Build history of the part. All positions in model axes, mm. A direction names the side the tool comes from. Coordinates: 2 decimals unless noted, no trailing zeros. Write each loop counter-clockwise with the first axis right and the second up, starting at its lowest first coordinate (ties: lowest second). Pieces come first, ordered by that corner, then holes.
```python
from build123d import *

# Parameters (mm, degrees)
F1_DEPTH = 5
F2_R     = 2.4
F2_R_2   = 0.75
F3_DEPTH = 2
F4_W     = 7
F4_H     = 3
F5_DEPTH = 3


with BuildPart() as f1:
    # F0 (on Right) → F1 (new body)
    with BuildSketch(Plane.YZ):
        with BuildLine():
            ThreePointArc((10, 30), (0, 40), (-10, 30))
            Line((-10, 30), (-10, 0))
            Line((-10, 0), (10, 0))
            Line((10, 0), (10, 30))
        make_face()
    extrude(amount=F1_DEPTH)

    # F2 (on face) → F3 (cut)
    with BuildSketch(Plane.YZ.offset(5)):
        with Locations((0, 30)):
            Circle(F2_R)
        with Locations((0, 30)):
            Circle(F2_R_2, mode=Mode.SUBTRACT)
    extrude(amount=-F3_DEPTH, mode=Mode.SUBTRACT)

    # F4 (on face) → F5 (join)
    with BuildSketch(Plane.YZ.offset(5)):
        with Locations((-6.5, -1.5)):
            Rectangle(F4_W, F4_H)
        with Locations((6.5, -1.5)):
            Rectangle(F4_W, F4_H)
    extrude(amount=-F5_DEPTH)


solid = f1.part
```
1. 3-axis set-ups, long thin cutter, end or side, ignore diameter. For faces 1 (the face through (4, -3, -2)), 2 (the face through (4.014, -0.098, 30.744)), 3 (the face through (5, 0, 19)), 4 (the face through (2, 6, -1)): which of +Z, -Z, +X, -X, +Y, -Y reach the whole face in a straight line?
Computed values:
face 1: -Z, +X, -X
face 2: +X
face 3: +Z, -Z, +X, +Y, -Y
face 4: -Z, -X, +Y, -Y
2. Saw through at B-B on y = 0. List the corners of the cut face in (x, z).
Computed values:
outline: (0, 0) - (5, 0) - (5, 27.6) - (3, 27.6) - (3, 29.25) - (5, 29.25) - (5, 30.75) - (3, 30.75) - (3, 32.4) - (5, 32.4) - (5, 40) - (0, 40) - close
3. Probe line 1 along Z through (x, y) = (3.2, 1.5); line 2 along Z through (x, y) = (4.1, 6.5); line 3 along Z through (x, y) = (1.25, 9). List the from-to ranges inside material, lowest first.
Computed values:
line 1: z = 0 to 28.13, 31.87 to 39.89
line 2: z = -3 to 37.6
line 3: z = 0 to 34.36
4. Saw through at D-D on z = 37.5. List the corners of the cut face in (x, y), plus the area to 3 significant figures.
Computed values:
outline: (0, -6.61) - (5, -6.61) - (5, 6.61) - (0, 6.61) - close
area: 66.1 mm2
5. Saw through at C-C on x = 0.5. List the corners of the cut face in (y, z), plus the area to 3 significant figures.
Computed values:
outline: (-10, 0) - (10, 0) - (10, 30) arc R10 ccw to (-10, 30) - close
area: 757 mm2
6. Saw through at A-A on x = 3.7. List the corners of the cut face in (y, z).
Computed values:
outline: (-10, -3) - (-3, -3) - (-3, 0) - (3, 0) - (3, -3) - (10, -3) - (10, 30) arc R10 ccw to (-10, 30) - close; circle Ø1.5 at (0, 30); hole circle Ø4.8 at (0, 30)
7. Flat gauge pins, fed straight in: pin 1 (6 mm diameter, centred on y = -1.5, z = 21.5, fed in from -X); pin 2 (0.9 mm diameter, centred on y = -7, z = -1.5, fed in from -X); pin 3 (1.5 mm diameter, centred on x = 2.5, y = 2, fed in from -Z). Where does each tip first touch, or does it go through?
Computed values:
pin 1: stops at x = 0
pin 2: stops at x = 2
pin 3: stops at z = 0
8. Mould opens along Z. For faces 5 (the face through (4.014, -0.52, 27.657)), 6 (the face through (2, 0, 40)), 7 (the face through (4, -7, -3)), 8 (the face through (2, -7, -1)) say: +Z half, -Z half, draft (parallel to the pull), parting line (faces both ways), or undercut.
Computed values:
face 5: undercut
face 6: +Z half
face 7: -Z half
face 8: draft
